Model file for the job. Use its own axes, mm. Face numbers are marked on the shaded views. A direction names the side the tool comes from. Give positions to 0.01 mm unless a question says otherwise; leave off trailing zeros. Write each loop counter-clockwise with the first axis right and the second up, starting at its lowest first coordinate (ties: lowest second). Pieces come first, ordered by that corner, then holes.
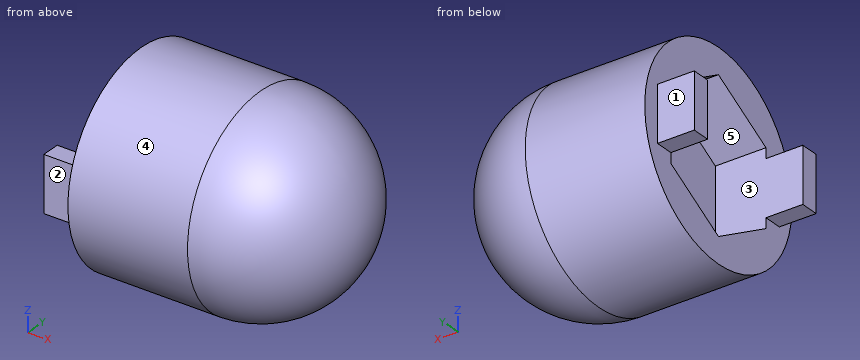
```python
from build123d import *

# Parameters (mm, degrees)
CUT_EXTRUDE1_DEPTH  = 2.75
SKETCH5_W           = 3
SKETCH5_H           = 1
BOSS_EXTRUDE2_DEPTH = 2


with BuildPart() as part:
    # Sketch1 → Revolve1 (revolve)
    with BuildSketch(Plane.XY, mode=Mode.PRIVATE) as revolve1_sk:
        with BuildLine():
            Line((0, 0), (12, 0))
            ThreePointArc((12, 0), (10.389087297, -3.889087297), (6.5, -5.5))
            Line((6.5, -5.5), (0, -5.5))
            Line((0, -5.5), (0, 0))
        make_face()
    revolve(revolve1_sk.sketch.rotate(Axis((0, 0, 0), (1, 0, 0)), 270), axis=Axis((0, 0, 0), (1, 0, 0)))

    # Sketch2 → Cut-Extrude1 (cut)
    with BuildSketch(Plane.ZY):
        Polygon((2.050748156, 3.552), (-2.050748156, 3.552), (-4.101496312, 0), (-2.050748156, -3.552), (2.050748156, -3.552), (4.101496312, 0), align=None)
    extrude(amount=-CUT_EXTRUDE1_DEPTH, mode=Mode.SUBTRACT)

    # Sketch5 → Boss-Extrude2 (add)
    with BuildSketch(Plane.ZY):
        with Locations((0, 4.052)):
            Rectangle(SKETCH5_W, SKETCH5_H)
        with Locations((0, -4.052)):
            Rectangle(SKETCH5_W, SKETCH5_H)
    extrude(amount=BOSS_EXTRUDE2_DEPTH)


solid = part.part
```
1. Pin check, flat tips, straight feed: P1, Ø0.8, axis at x = -1, y = -4, coming from the -Z side; P2, Ø1, axis at y = -3, z = -4, coming from the +X side; P3, Ø1.5, axis at x = 10.5, z = 0, coming from the -Y side. Stop position of each tip, or through.
Calculated:
P1: stops at z = -1.5
P2: stops at x = 9.66
P3: stops at y = -4.44
2. Slice it at B-B, the plane z = 0. Write the cut outline in (x, y), and give its area (3 significant figures).
Calculated:
outline: (-2, -4.55) - (0, -4.55) - (0, -5.5) - (6.5, -5.5) arc R5.5 ccw to (6.5, 5.5) - (0, 5.5) - (0, 4.55) - (-2, 4.55) - (-2, 3.55) - (2.75, 3.55) - (2.75, -3.55) - (-2, -3.55) - close
area: 103 mm2
3. Which spindle directions (+Z, -Z, +X, -X, +Y, -Y) get a long thin tool onto all of the face, cutting with end or side? Do the marked faces 4 and 5. Say none if no direction does.
Calculated:
face 4: +X, -X
face 5: -X
4. Probe probe 1 along Y at (x, z) = (2, 4); probe 2 along X at (y, z) = (1, 0); probe 3 along Z at (x, y) = (10.75, 2). List the from-to ranges inside material, lowest first.
Calculated:
probe 1: y = -3.77 to -0.18, 0.18 to 3.77
probe 2: x = 2.75 to 11.91
probe 3: z = -2.86 to 2.86
5. Slice it at A-A, the plane x = 1. Write the cut outline in (y, z).
Calculated:
outline: circle Ø11 at (0, 0); hole (-3.55, -2.05) - (0, -4.1) - (3.55, -2.05) - (3.55, 2.05) - (0, 4.1) - (-3.55, 2.05) - close
6. Pull direction Y, two halves, no side cores. Call the marked faces 1, 2 and 3: +Y half, -Y half, draft (parallel to the pull), parting line (faces both ways), or undercut.
Calculated:
face 1: +Y half
face 2: -Y half
face 3: undercut
7. Slice it at D-D, the plane y = 5. Write the cut outline in (x, z).
Calculated:
outline: (0, -2.29) - (6.5, -2.29) arc R2.29 ccw to (6.5, 2.29) - (0, 2.29) - close
8. Slice it at C-C, the plane x = 4.75. Write the cut outline in (y, z).
Calculated:
outline: circle Ø11 at (0, 0)
